Input: part model. Units: mm. Frame: model coordinates. A direction names the side the tool comes from. Round coordinates to 2 decimals unless told otherwise and drop trailing zeros. Loops run counter-clockwise (first coordinate to the right, second up) from the corner with the lowest first, then second, coordinate; pieces in that order, holes last. Notation, with made-up numbers: (-29, 35) - (-19, 35) arc R28 ccw to (-19, 53) - close; hole circle Ø9 at (38, 84). An arc over 180 degrees is marked (long way). Use CSV: the item, a comma, the result in double quotes. Start each with the question number.
1. Cut plane B-B (y = 5.04). Return loops of the section in (x, z).
2. Pin query (flat end, axial travel): P1, Ø4, axis at x = 365, z = 482.5, coming from the +Y side; P2, Ø4, axis at y = 5, z = 454.5, coming from the +X side; P3, Ø3, axis at x = 376.5, y = 15.5, coming from the -Z side. Return the tip coordinate at first contact, or that it passes through.
3. Cut plane C-C (x = 395). Return loops of the section in (y, z), and give its area (3 significant figures).
4. Material intervals for probe 1 along Z at (x, y) = (377.5, 18.5); probe 2 along Y at (x, z) = (394, 447); probe 3 along Y at (x, z) = (368.5, 453), sorted ascending. Write a range as from..to.
5. Cut plane A-A (z = 454.5). Return loops of the section in (x, y).
6. Pull-direction query (Z, two-part tool) for faces 1 (the flat face through (377.728, -3.013, 502.919)), 2 (the flat face through (380.768, 12, 504)), 3 (the flat face through (366, 3, 456.09)); classes: +Z half, -Z half, draft (parallel to the pull), parting line (faces both ways), or undercut.
7. Cut plane D-D (x = 384.5). Return loops of the section in (y, z), and give its area (3 significant figures).
8. Access query for faces 4 (the flat face through (378, 12, 505.725)), 5 (the flat face through (374.768, 12, 504)), 6 (the flat face through (372.54, 5, 482)). Directions: +Z, -Z, +X, -X, +Y, -Y. A direction counts if a zero-diameter tool reaches every point of the face in a straight line with its end or side. Return the directions, or none.
```python
from build123d import *

# Parameters (mm, degrees)
SKETCH1_W                = 50
SKETCH1_H                = 66.947148402
SKETCH1_R                = 10
SKETCH1_W_2              = 10
SKETCH1_H_2              = 5
BOSS_EXTRUDE1_DEPTH      = 2.54
BOSS_EXTRUDE2_DEPTH      = 5
BOSS_EXTRUDE2_DEPTH_BACK = 2.54
SKETCH2_W                = 10
SKETCH2_H                = 5
SKETCH3_R                = 2.05
CUT_EXTRUDE1_DEPTH       = 41
SKETCH4_W                = 6
SKETCH4_H                = 2.904570335
BOSS_EXTRUDE3_DEPTH      = 20
SKETCH5_R                = 1.5
CUT_EXTRUDE2_DEPTH       = 20
SKETCH6_W                = 5.734558075
SKETCH6_H                = 6.4250327
BOSS_EXTRUDE4_DEPTH      = 10
DRAFT1_ANGLE             = -1
DRAFT2_START             = 371.742315671
DRAFT2_OUTLINE_W         = 10
DRAFT2_OUTLINE_H         = 6.426011413
DRAFT2_DEPTH             = 1.257684329
DRAFT3_START             = -2
DRAFT3_OUTLINE_W         = 9
DRAFT3_OUTLINE_H         = 10
DRAFT3_DEPTH             = 0.836252296
DRAFT4_ANGLE             = 1
CHAMFER1_SIZE            = 10
CHAMFER1_SIZE_2          = 10.179201911
FILLET2_R                = 0.2


with BuildPart() as part:
    # Sketch1 → Boss-Extrude1 (new body)
    with BuildSketch(Plane(origin=(0, 0, 0), x_dir=(1, 0, 0), z_dir=(0, 1, 0))):
        with Locations((377.767738439, -474.515341444)):
            Rectangle(SKETCH1_W, SKETCH1_H)
        with Locations(Location((388.753012651, -492.770944419, 0), (0, 0, 270))):
            Circle(SKETCH1_R, mode=Mode.SUBTRACT)
        with Locations((367.539675888, -481.590375858)):
            Rectangle(SKETCH1_W_2, SKETCH1_H_2, mode=Mode.SUBTRACT)
        with Locations((367.539675888, -453.590375858)):
            Rectangle(SKETCH1_W_2, SKETCH1_H_2, mode=Mode.SUBTRACT)
    extrude(amount=BOSS_EXTRUDE1_DEPTH)

    # Sketch2 → Boss-Extrude2 (add, two sides: drawn at the far end of the back side and taken through both)
    with BuildSketch(Plane(origin=(0, 2.54, 0), x_dir=(1, 0, 0), z_dir=(0, 1, 0)).offset(-BOSS_EXTRUDE2_DEPTH_BACK)):
        with Locations((367.539675888, -453.590375858)):
            Rectangle(SKETCH2_W, SKETCH2_H)
        with Locations((367.539675888, -481.590375858)):
            Rectangle(SKETCH2_W, SKETCH2_H)
    extrude(amount=BOSS_EXTRUDE2_DEPTH + BOSS_EXTRUDE2_DEPTH_BACK)

    # Sketch3 → Cut-Extrude1 (cut)
    with BuildSketch(Plane(origin=(0, 0, 451.090375858), x_dir=(-1, 0, 0), z_dir=(0, 0, -1))):
        with Locations((-367.539675888, 5.04)):
            Circle(SKETCH3_R)
    extrude(amount=-CUT_EXTRUDE1_DEPTH, mode=Mode.SUBTRACT)

    # Sketch4 → Boss-Extrude3 (add)
    with BuildSketch(Plane(origin=(0, 2.54, 0), x_dir=(1, 0, 0), z_dir=(0, 1, 0))):
        with Locations((377.767738439, -504.273195611)):
            Rectangle(SKETCH4_W, SKETCH4_H)
    extrude(amount=BOSS_EXTRUDE3_DEPTH)

    # Sketch5 → Cut-Extrude2 (cut)
    with BuildSketch(Plane.XY.offset(505.725480778)):
        with Locations((377.767738439, 20.423645689)):
            Circle(SKETCH5_R)
    extrude(amount=-CUT_EXTRUDE2_DEPTH, mode=Mode.SUBTRACT)

    # Sketch6 → Boss-Extrude4 (add)
    with BuildSketch(Plane(origin=(0, 0, 0), x_dir=(-1, 0, 0), z_dir=(0, -1, 0))):
        with Locations((-377.767738439, -503.005882789)):
            Rectangle(SKETCH6_W, SKETCH6_H)
    extrude(amount=BOSS_EXTRUDE4_DEPTH)

    # Draft1
    draft1_faces = [part.faces().sort_by_distance(p)[0] for p in [
        (374.900459401, -5, 503.005882789),
    ]]
    draft(draft1_faces, Plane(origin=(374.900459401, -10, 506.218399139), x_dir=(1, 0, 0), z_dir=(0, 0, 1)), DRAFT1_ANGLE)

    # Draft2: read off the stored shape, not the designer's step
    # Draft2 outline → Draft2 (cut)
    with BuildSketch(Plane(origin=(0, 0, 0), x_dir=(0, 1, 0), z_dir=(0.9998476951563913, 0, -0.017452406437283505)).offset(DRAFT2_START)):
        with Locations((-5, 509.571290948)):
            Rectangle(DRAFT2_OUTLINE_W, DRAFT2_OUTLINE_H)
    extrude(amount=DRAFT2_DEPTH, mode=Mode.SUBTRACT)

    # Draft3: read off the stored shape, not the designer's step
    # Draft3 outline → Draft3 (cut)
    with BuildSketch(Plane(origin=(0, 0, 0), x_dir=(1, 0, 0), z_dir=(0, 0.9998476951563913, 0.017452406437283505)).offset(DRAFT3_START)):
        with Locations((377.5, -503)):
            Rectangle(DRAFT3_OUTLINE_W, DRAFT3_OUTLINE_H)
    extrude(amount=DRAFT3_DEPTH, mode=Mode.SUBTRACT)

    # Draft4
    draft4_faces = [part.faces().sort_by_distance(p)[0] for p in [
        (377.767738439, -5, 506.218399139),
    ]]
    draft(draft4_faces, Plane(origin=(374.900459401, -10, 506.218399139), x_dir=(0, 0.017452406437283553, -0.9998476951563913), z_dir=(0, -0.9998476951563913, -0.017452406437283553)), DRAFT4_ANGLE)

    # Chamfer1
    # the kernel refuses this chamfer: 10.179201911, 10 mm, written as the material it takes off along each edge
    with BuildSketch(Plane(origin=(348.822826033, -9.887850637, 499.793366439), x_dir=(0, 1, 0), z_dir=(1, 0, 0))) as chamfer1_piece_1_section:
        Polygon((CHAMFER1_SIZE, 0), (-CHAMFER1_SIZE_2 * 0.0174524064368, CHAMFER1_SIZE_2 * 0.999847695128), (0, 0), align=None)
    chamfer1_piece_1 = extrude(amount=57.889824811, mode=Mode.PRIVATE)
    chamfer1_piece_1 = split(chamfer1_piece_1, bisect_by=Plane(origin=(348.822826033, 0, 499.793366439), z_dir=(0, -1, 0)), keep=Keep.TOP, mode=Mode.PRIVATE)
    add(chamfer1_piece_1, mode=Mode.SUBTRACT)

    # Fillet2
    fillet2_edges = [part.edges().sort_by_distance(p)[0] for p in [
        (377.767738438, -6.437295713, 506.342811514),
    ]]
    fillet(fillet2_edges, radius=FILLET2_R)


solid = part.part
```
Established:
1,outline,"(362.54, 451.09) - (365.49, 451.09) - (365.49, 456.09) - (362.54, 456.09) - close; (362.54, 479.09) - (365.49, 479.09) - (365.49, 484.09) - (362.54, 484.09) - close; (369.59, 451.09) - (372.54, 451.09) - (372.54, 456.09) - (369.59, 456.09) - close; (369.59, 479.09) - (372.54, 479.09) - (372.54, 484.09) - (369.59, 484.09) - close; (374.77, 502.82) - (380.77, 502.82) - (380.77, 505.73) - (374.77, 505.73) - close"
2,P1,"stops at y = 7.54"
2,P2,"stops at x = 372.54"
2,P3,"stops at z = 502.82"
3,outline,"(0, 441.04) - (2.54, 441.04) - (2.54, 484.96) - (0, 484.96) - close; (0, 500.58) - (2.54, 500.58) - (2.54, 507.99) - (0, 507.99) - close"
3,area,"130 mm2"
4,probe 1,"z = 502.82..505.73"
4,probe 2,"y = 0..2.54"
4,probe 3,"y = 0..3.23, 6.85..7.54"
5,outline,"(352.77, 0) - (402.77, 0) - (402.77, 2.54) - (372.54, 2.54) - (372.54, 7.54) - (362.54, 7.54) - (362.54, 2.54) - (352.77, 2.54) - close; hole circle Ø4.1 at (367.54, 5.04)"
6,face 1,"-Z half"
6,face 2,"draft"
6,face 3,"undercut"
7,outline,"(0, 441.04) - (2.54, 441.04) - (2.54, 483.72) - (0, 483.72) - close; (0, 501.82) - (2.54, 501.82) - (2.54, 507.99) - (0, 507.99) - close"
7,area,"124 mm2"
8,face 4,"+Z, +X, -X, +Y"
8,face 5,"+Z, -Z, -X, +Y"
8,face 6,"+Z, -Z, +X, +Y"
